Work out the finished part from the listing and answer in its coordinate system (mm). Face numbers are marked on the shaded views. A direction names the side the tool comes from. Coordinates: 2 decimals unless noted, no trailing zeros. Write each loop counter-clockwise with the first axis right and the second up, starting at its lowest first coordinate (ties: lowest second). Pieces come first, ordered by that corner, then holes. Notation, with made-up numbers: (5.5, 28.5) - (45.5, 28.5) arc R15 ccw to (45.5, 43.5) - close; hole circle Ø6 at (3.5, 64). An arc over 180 degrees is marked (long way). Answer as a JSON object with one key per item and string values. Group by question number.
Autodesk Inventor part; units mm, degrees
ref_plane "YZ Plane" through (0, 0, 0) normal (1, 0, 0) x (0, 1, 0)
ref_plane "XZ Plane" through (0, 0, 0) normal (0, 1, 0) x (-1, 0, 0)
ref_plane "XY Plane" through (0, 0, 0) normal (0, 0, 1) x (1, 0, 0)
sketch "Sketch1" plane through (0, 0, 0) normal (0, 0, 1) x (1, 0, 0)
  circle A0 centre (0, 0) radius 10
  dimension "d0" = 20
extrude "Extrusion1" add sketch "Sketch1" along normal blind 10
sketch "Sketch2" plane through (0, 0, 10) normal (0, 0, 1) x (1, 0, 0)
  circle A0 centre (0, 0) radius 3
  dimension "d3" = 6
extrude "Extrusion2" add sketch "Sketch2" along normal blind 12
sketch "Sketch3" plane through (0, 0, 22) normal (0, 0, 1) x (1, 0, 0)
  circle A0 centre (0, 0) radius 9
  dimension "d6" = 18
extrude "Extrusion3" add sketch "Sketch3" along normal blind 3
sketch "Sketch4" plane through (0, 0, 25) normal (0, 0, 1) x (1, 0, 0)
  circle A0 centre (0, 6) radius 1.5
  circle A1 centre (4.2426, 4.2426) radius 0.75
  line L0 (0, 0) -> (0, 14.9818) construction
  line L1 (0, 0) -> (4.2426, 4.2426) construction
  dimension "d9" = 3
  dimension "d10" = 1.5
  dimension "d11" = 0
  dimension "d12" = 6
  dimension "d13" = 45
  dimension "d14" = 0
  dimension "d15" = 6
  dimension "d16" = 0
extrude "Extrusion4" add sketch "Sketch4" along normal blind 3 contours A0
extrude "Extrusion5" cut sketch "Sketch4" against normal blind 3 contours A1
fillet "Fillet1" radius 1 1 edges at (-1.5, 6, 28)
pattern_circular "Circular Pattern1" count 4 over 360 about axis through (0, 0, 22) along (0, 0, 1) of "Extrusion4", "Fillet1", "Extrusion5"
properties part number "Motor1Gear"
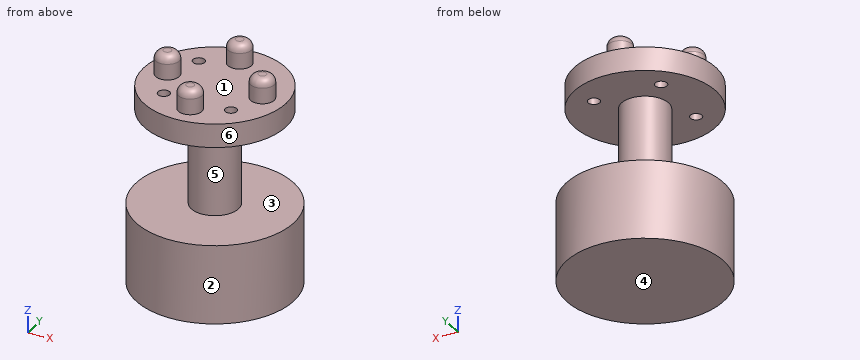
Q1. A tool of negligible diameter and unlimited length cuts with its end or side. For the marked faces 5 and 6, from which of +Z, -Z, +X, -X, +Y, -Y can it reach the whole face along a straight path? Write none if from no direction.
Q2. Flat-ended cylindrical pins translate along their axes: pin 1 Ø4 at (x, z) = (-5.5, 8) entering from +Y; pin 2 Ø3 at (x, y) = (4.5, 7) entering from +Z; pin 3 Ø8 at (x, z) = (8, 5) entering from -Y. Find the tip coordinate at first contact, or state that the pin passes through.
Q3. Section B-B on z = 15 is taken. Determine the outline of the cut face in (x, y).
Q4. Section A-A on x = -8 is taken. Determine the outline of the cut face in (y, z), plus the area to 3 significant figures.
Q5. For a pull along Z with two mould halves and no side action, classify the marked faces 1, 2, 3 and 4 as +Z half, -Z half, draft (parallel to the pull), parting line (faces both ways), or undercut.
Q6. Consider L1, parallel to Z at x = -6.25, y = -3; L2, parallel to Z at x = -9, y = -2.25; L3, parallel to Z at x = -1.25, y = -5.75. Determine where each line is inside the solid, lowest interval first. Write a range as from..to.
Q7. Section C-C on z = 6 is taken. Determine the outline of the cut face in (x, y).
Numbers:
{
 "1": {"face 5": "none", "face 6": "+Z"},
 "2": {"pin 1": "stops at y = 9.37", "pin 2": "stops at z = 25", "pin 3": "stops at y = -9.17"},
 "3": {"outline": "circle Ø6 at (0, 0)"},
 "4": {"outline": "(-6, 0) - (6, 0) - (6, 10) - (-6, 10) - close; (-4.12, 22) - (4.12, 22) - (4.12, 25) - (-4.12, 25) - close", "area": "145 mm²"},
 "5": {"face 1": "+Z half", "face 2": "draft", "face 3": "undercut", "face 4": "-Z half"},
 "6": {"L1": "z = 0..10, 22..25", "L2": "z = 0..10", "L3": "z = 0..10, 22..27.63"},
 "7": {"outline": "circle Ø20 at (0, 0)"}
}
